Answer from the drawing. Dimensions are ordinates in mm from the lowest x, y and z of the part. A direction names the side the tool comes from. Give positions to 0.01 mm unless a question says otherwise; leave off trailing zeros. Order: outer loops, then holes, each group sorted by start corner. A loop starts at its lowest first (then second) coordinate and runs counter-clockwise, first axis right, second up. Notation, with made-up numbers: M -8.5,44.25 L 7.5,44.25 A9 ccw 7.5,52.25 Z; hole C -17,-38.75 d5. An arc over 180 degrees is marked long. One line per item, written item: value.
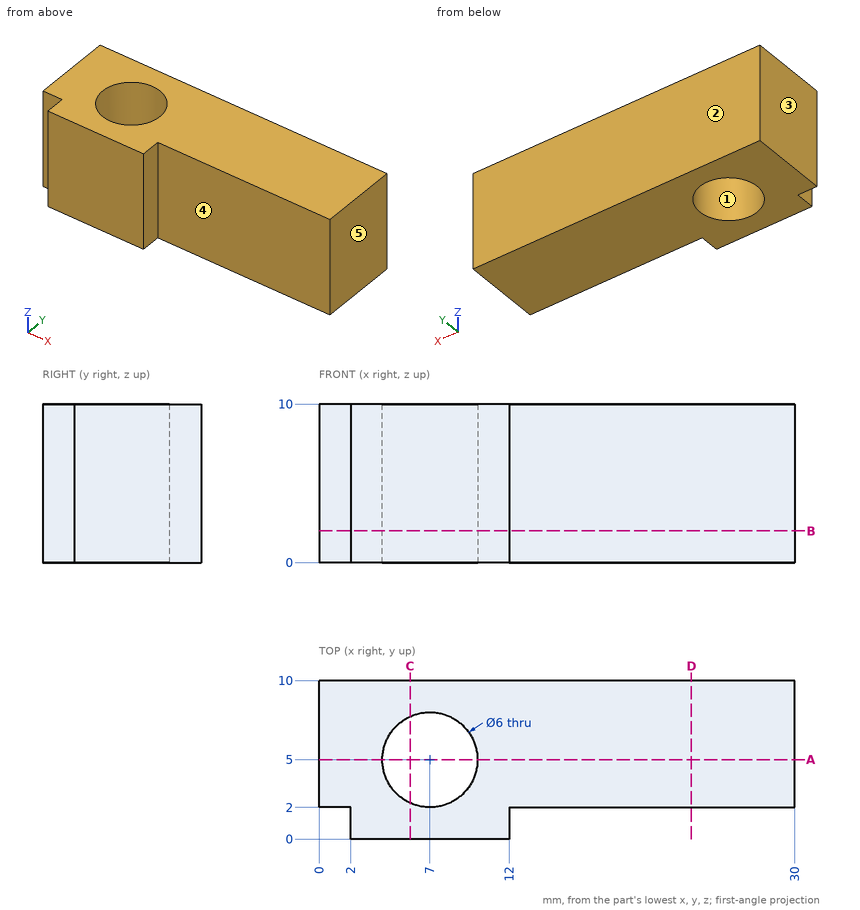
(1) Section C-C, the plane x = 5.75 is taken. Give the vertices of the cut face in (y, z).
Findings:
outline: M 0,0 L 2.27,0 L 2.27,10 L 0,10 Z; M 7.73,0 L 10,0 L 10,10 L 7.73,10 Z
(2) Find the intervals of material crossed by probe 1 along Y at (x, z) = (7, 5.25); probe 2 along Y at (x, z) = (24, 6); probe 3 along Y at (x, z) = (9.25, 1), in increasing order. Write a range as from..to.
Findings:
probe 1: y = 0..2, 8..10
probe 2: y = 2..10
probe 3: y = 0..3.02, 6.98..10
(3) Section D-D, the plane x = 23.5 is taken. Give the vertices of the cut face in (y, z).
Findings:
outline: M 2,0 L 10,0 L 10,10 L 2,10 Z
(4) Section A-A, the plane y = 5 is taken. Give the vertices of the cut face in (x, z).
Findings:
outline: M 0,0 L 4,0 L 4,10 L 0,10 Z; M 10,0 L 30,0 L 30,10 L 10,10 Z
(5) Which of the six approach directions +Z, -Z, +X, -X, +Y, -Y give full straight-line access (tool end or side, diameter ignored) to the marked faces 4 and 5?
Findings:
face 4: +Z, -Z, +X, -Y
face 5: +Z, -Z, +X, +Y, -Y
(6) Determine the mould class of the marked faces 1, 2 and 3 for opening direction Y: pulls with the +Y half, pulls with the -Y half, needs draft (parallel to the pull), parting line crosses it, or undercut.
Findings:
face 1: undercut
face 2: pulls with the +Y half
face 3: needs draft
(7) Given P1, Ø1.6, axis at x = 1, z = 4, coming from the -Y side; P2, Ø1, axis at y = 0.5, z = 5.5, coming from the +X side; P3, Ø0.6, axis at y = 1, z = 5, coming from the -X side, each flat-ended and moving along its own axis, determine where each tip first touches the part or whether it passes through.
Findings:
P1: stops at y = 2
P2: stops at x = 12
P3: stops at x = 2
(8) Section B-B, the plane z = 2 is taken. Give the vertices of the cut face in (x, y).
Findings:
outline: M 0,2 L 2,2 L 2,0 L 12,0 L 12,2 L 30,2 L 30,10 L 0,10 Z; hole C 7,5 d6
